Geometry: final body of the model. Coordinates: model frame, mm. A direction names the side the tool comes from. Coordinates: 2 decimals unless noted, no trailing zeros. Write each loop counter-clockwise with the first axis right and the second up, starting at its lowest first coordinate (ties: lowest second). Pieces come first, ordered by that corner, then holes. Notation, with made-up numbers: (83, 89.25) -> (104, 89.25) arc R20 cw to (104, 125.25) -> close; hole circle Ø1 at (11.25, 87). An arc over 180 degrees is marked (long way). One line per item, written item: value.
Autodesk Inventor part; units mm, degrees
ref_plane "YZ Plane" through (0, 0, 0) normal (1, 0, 0) x (0, 1, 0)
ref_plane "XZ Plane" through (0, 0, 0) normal (0, 1, 0) x (-1, 0, 0)
ref_plane "XY Plane" through (0, 0, 0) normal (0, 0, 1) x (1, 0, 0)
sketch "Sketch1" plane through (0, 0, 0) normal (0, 0, 1) x (1, 0, 0)
  line L0 (5.4993, 0) -> (2.7496, -4.7625)
  line L1 (2.7496, -4.7625) -> (-2.7496, -4.7625)
  line L2 (-2.7496, -4.7625) -> (-5.4993, 0)
  line L3 (-5.4993, 0) -> (-2.7496, 4.7625)
  line L4 (-2.7496, 4.7625) -> (2.7496, 4.7625)
  line L5 (2.7496, 4.7625) -> (5.4993, 0)
  circle A0 centre (0, 0) radius 0.0127
  dimension "d0" = 9.525
  dimension "d6" = 0.0254
extrude "Extrusion2" add sketch "Sketch1" along normal mid plane 114.3
sketch "Sketch4" plane through (0, 0, -57.15) normal (0, 0, -1) x (-1, 0, 0)
  circle A0 centre (0, 0) radius 0.0127
  circle A1 centre (0, 0) radius 12.7
  dimension "d10" = 25.4
extrude "Extrusion4" add sketch "Sketch4" against normal blind 19.05
thicken "Reduce Hex Shaft" operation add thickness 0.127 both sides no extend neighbours yes toward (0, -1, 0) faces at (0.9165, 4.7625, -6.35) (4.5827, 1.5875, -6.35) (3.6662, -3.175, -6.35) (-3.6662, 3.175, -6.35) (-4.5827, -1.5875, -6.35) (-0.9165, -4.7625, -6.35)
sketch "Sketch5" plane through (0, 0, -38.1) normal (0, 0, 1) x (1, 0, 0)
  circle A0 centre (0, 0) radius 6.35
  dimension "d15" = 12.7
extrude "Extrusion5" add sketch "Sketch5" along normal blind 6.35
thicken "Reduce Base Bushing" operation add thickness 0.127 both sides no extend neighbours yes toward (-0.9967573, 0.0804666, 0) faces at (6.3294, -0.511, -33.8667)
equation "\"d0\" = hexSize"
equation "\"d4\" = length"
equation "\"d13\" = printOffset"
equation "\"d14\" = printOffset"
equation "\"d15\" = bushingForBaseHole"
equation "\"d16\" = sideOfBase"
equation "\"d20\" = printOffset"
equation "\"d21\" = printOffset"
equation "\"hexSize\" = 9.525"
equation "\"length\" = 114.3"
equation "\"printOffset\" = 0.127"
equation "\"bushingForBaseHole\" = 12.7"
equation "\"sideOfBase\" = 6.35"
properties part number "3_8x4_5-inchHexShaft" material "PC/ABS Plastic"
(1) Section D-D (x = -7.5). Return the cut outline in (y, z).
Responses:
outline: (-10.25, -57.15) -> (10.25, -57.15) -> (10.25, -38.1) -> (-10.25, -38.1) -> close
(2) Line query: line 1 (Z direction, x = -9.5, y = 4.5); line 2 (Y direction, x = 1.5, z = 28.5); line 3 (Y direction, x = -3.25, z = 4.5). Output: solid intervals per line, ascending. Write a range as [from, to].
Responses:
line 1: z = [-57.15, -38.1]
line 2: y = [-4.64, 4.64]
line 3: y = [-3.64, 3.64]
(3) Reachability of faces 1 (the flat face through (-3.996, -2.35, 12.078)), 2 (the flat face through (0, -4.636, 12)), 3 (the flat face through (0, 4.636, 12)), 4 (the flat face through (4.03, -2.29, 12.08)), 5 (the flat face through (-3, 6, -38.1)) from +Z, -Z, +X, -X, +Y, -Y: full face, straight path, thin tool, end or side. Return the list, or none.
Responses:
face 1: +Z, -X, -Y
face 2: +Z, +X, -X, -Y
face 3: +Z, +X, -X, +Y
face 4: +Z, +X, -Y
face 5: +Z
(4) Section B-B (y = -3.25). Return the cut outline in (x, z).
Responses:
outline: (-12.28, -57.15) -> (12.28, -57.15) -> (12.28, -38.1) -> (5.31, -38.1) -> (5.31, -31.75) -> (3.48, -31.75) -> (3.48, 57.15) -> (-3.48, 57.15) -> (-3.48, -31.75) -> (-5.31, -31.75) -> (-5.31, -38.1) -> (-12.28, -38.1) -> close
(5) First-contact query: pin 1 (12 mm diameter, centred on y = -6.5, z = 20.5, fed in from -X); pin 2 (10 mm diameter, centred on x = 3, y = -5.5, fed in from +Z); pin 3 (4.5 mm diameter, centred on x = -1.5, z = 5, fed in from -Y); pin 4 (6 mm diameter, centred on y = 8, z = -2, fed in from +X). Flat tips, straight axial feed; report the tip coordinate or a pass-through.
Responses:
pin 1: stops at x = -5.06
pin 2: stops at z = 57.15
pin 3: stops at y = -4.64
pin 4: passes through
